```python
from build123d import *

# Parameters (mm, degrees)
F3_R     = 2.5
F4_DEPTH = 56.9
F5_R     = 2.5
F6_DEPTH = 26.75
F7_R     = 2.75
F8_DEPTH = 25


with BuildPart() as f2:
    # F0 (on Front) → F2 (revolve)
    with BuildSketch(Plane.XZ):
        Polygon((6.011957, 27), (-23.288043, 27), (-23.288043, 5), (9.441957, 5), (9.441957, 13.98), (22.711957, 13.98), (22.711957, 27.18), (19.511957, 27.18), (19.511957, 23), (9.511957, 23), (9.511957, 30.5), (6.011957, 30.5), align=None)
    revolve(axis=Axis((-13.926744, 0, 0), (-1, 0, 0)))

    # F3 (on Front) → F4 (cut, symmetric)
    with BuildSketch(Plane.XZ):
        with Locations((-3.348043, 0)):
            Circle(F3_R)
    extrude(amount=F4_DEPTH, both=True, mode=Mode.SUBTRACT)

    # F5 (on face) → F6 (cut)
    with BuildSketch(Plane(origin=(-23.288043, 0, 0), x_dir=(0, -1, 0), z_dir=(-1, 0, 0))):
        with Locations((0, -11.75)):
            Circle(F5_R)
        with Locations((0, 11.75)):
            Circle(F5_R)
    extrude(amount=-F6_DEPTH, mode=Mode.SUBTRACT)

    # F7 (on Front) → F8 (cut)
    with BuildSketch(Plane.XZ):
        with Locations((14.511957, 0)):
            Circle(F7_R)
    extrude(amount=-F8_DEPTH, mode=Mode.SUBTRACT)


solid = f2.part
```
Here's how the part is built. I have some questions about the finished solid (model axes, mm). A direction names the side the tool comes from. Coordinates: 2 decimals unless noted, no trailing zeros. Write each loop counter-clockwise with the first axis right and the second up, starting at its lowest first coordinate (ties: lowest second). Pieces come first, ordered by that corner, then holes. Notation, with made-up numbers: (10.25, 50) -> (38.25, 50) arc R20 ccw to (38.25, 55) -> close; hole circle Ø2 at (-30.75, 12.25). An arc over 180 degrees is marked (long way). Use a Markdown table: item, result. Add a question column.
(1) If we section it at D-D, the plane z = 0: State how many separate pieces and enclosed holes the cut face has, and give its area (3 significant figures).
(2) I'm going to push flat-ended pins straight in: P1, Ø8, axis at x = -3.35, z = 0, coming from the -Y side; P2, Ø4, axis at y = 0, z = -11.5, coming from the -X side; P3, Ø10, axis at x = -7.5, z = 4, coming from the +Y side. Where does each tip first touch, or does it pass through?
(3) For faces 4 (the cylindrical face through (14.442, 22.804, -2.994)), 5 (the cylindrical face through (16.17, -13.648, -3.031)), 6 (the cylindrical face through (-10.1, 0.5, 9.3)), which set-ups out of +Z, -Z, +X, -X, +Y, -Y let a thin tool reach every point of the face, with its end or its side?
(4) Please list where these lines run through material, in increasing order: line 1 (X direction, y = 19.5, z = 0); line 2 (X direction, y = -19.25, z = 0); line 3 (X direction, y = 16, z = -24).
(5) If we section it at C-C, the plane x = -5: Write out the boundary of the cut face in (y, z), and give its area (3 significant figures).
(6) If we section it at B-B, the plane y = 24.5: Write out the boundary of the cut face in (x, z).
(7) We'd pull the mould along Z, two halves only. Please class faces 1 (the flat face through (9.512, 23, -4)), 2 (the cylindrical face through (7.737, -18.559, -24.204)), 3 (the cylindrical face through (-10.1, 0.5, -14.2)): +Z half, -Z half, draft (parallel to the pull), parting line (faces both ways), or undercut.
Outcome:
| question | item | result |
|---|---|---|
| 1 | separate pieces | 5 |
| 1 | enclosed holes | 0 |
| 1 | area | 1,460 mm^2 |
| 2 | P1 | stops at y = -27 |
| 2 | P2 | stops at x = 3.46 |
| 2 | P3 | stops at y = 27 |
| 3 | face 4 | none |
| 3 | face 5 | +X |
| 3 | face 6 | -X |
| 4 | line 1 | x = -23.29 to -5.85, -0.85 to 11.76, 17.26 to 22.71 |
| 4 | line 2 | x = -23.29 to -5.85, -0.85 to 22.71 |
| 4 | line 3 | x = 6.01 to 9.51 |
| 5 | outline | (-26.93, -1.88) arc R27 ccw to (26.93, -1.88) -> (4.63, -1.88) arc R5 cw to (-4.63, -1.88) -> close; (-26.93, 1.88) -> (-4.63, 1.88) arc R5 cw to (4.63, 1.88) -> (26.93, 1.88) arc R27 ccw to start; hole circle Ø5 at (0, -11.75); hole circle Ø5 at (0, 11.75) |
| 5 | area | 2,010 mm^2 |
| 6 | outline | (-23.29, -11.35) -> (6.01, -11.35) -> (6.01, -18.17) -> (9.51, -18.17) -> (9.51, 18.17) -> (6.01, 18.17) -> (6.01, 11.35) -> (-23.29, 11.35) -> close; (19.51, -11.77) -> (22.71, -11.77) -> (22.71, 11.77) -> (19.51, 11.77) -> close; hole circle Ø5 at (-3.35, 0) |
| 7 | face 1 | draft |
| 7 | face 2 | parting line |
| 7 | face 3 | undercut |
